```python
from build123d import *

# Parameters (mm, degrees)
BOSS_EXTRUDE1_DEPTH = 45
FILLET1_R           = 20
BOSS_EXTRUDE2_DEPTH = 19
BOSS_EXTRUDE3_DEPTH = 10
CUT_EXTRUDE2_REACH  = 92.422
SKETCH4_R           = 10
SKETCH4_R_2         = 5
SKETCH4_R_3         = 3
BOSS_EXTRUDE4_START = -9.5
SKETCH7_R           = 10
SKETCH7_R_2         = 5
BOSS_EXTRUDE4_DEPTH = 9.5


with BuildPart() as part:
    # Sketch1 → Boss-Extrude1 (new body)
    with BuildSketch(Plane.XY):
        Polygon((-53.872058339, 0), (-53.872058339, 13), (46.127941661, 13), (46.127941661, -4.908485857), (9.127941661, -4.908485857), (9.127941661, 0), align=None)
    extrude(amount=-BOSS_EXTRUDE1_DEPTH)

    # Fillet1
    fillet1_edges = [part.edges().sort_by_distance(p)[0] for p in [
        (46.127941661, 4.045757072, 0),
    ]]
    fillet(fillet1_edges, radius=FILLET1_R)

    # Sketch2 → Boss-Extrude2 (add)
    with BuildSketch(Plane(origin=(0, 0, -45), x_dir=(-1, 0, 0), z_dir=(0, 0, -1))):
        with BuildLine():
            Line((53.872058339, 13), (53.872058339, 51))
            ThreePointArc((53.872058339, 51), (34.872058339, 70), (15.872058339, 51))
            Line((15.872058339, 51), (15.872058339, 13))
            Line((15.872058339, 13), (53.872058339, 13))
        make_face()
        with BuildLine():
            Line((42.372058339, 51), (42.372058339, 32))
            ThreePointArc((42.372058339, 32), (34.872058339, 24.5), (27.372058339, 32))
            Line((27.372058339, 32), (27.372058339, 51))
            ThreePointArc((27.372058339, 51), (34.872058339, 58.5), (42.372058339, 51))
        make_face(mode=Mode.SUBTRACT)
    extrude(amount=-BOSS_EXTRUDE2_DEPTH)

    # Sketch3 → Boss-Extrude3 (add)
    with BuildSketch(Plane(origin=(0, 0, -45), x_dir=(-1, 0, 0), z_dir=(0, 0, -1))):
        Polygon((-46.127941661, 13), (16.803506509, 13), (18.329411345, 13), (18.329411345, 60.345631624), align=None)
    extrude(amount=-BOSS_EXTRUDE3_DEPTH)

    # Sketch4 → Cut-Extrude2 (cut, up to next)
    with BuildSketch(Plane(origin=(0, 13, 0), x_dir=(1, 0, 0), z_dir=(0, 1, 0)), mode=Mode.PRIVATE) as cut_extrude2_sk1:
        with Locations(Location((26.127941661, 20, 0), (0, 0, 270))):
            Circle(SKETCH4_R)
        with Locations((26.127941661, 20)):
            Circle(SKETCH4_R_2, mode=Mode.SUBTRACT)
    cut_extrude2_tool1 = extrude(cut_extrude2_sk1.sketch, amount=-CUT_EXTRUDE2_REACH, mode=Mode.PRIVATE) & part.part
    # Sketch4 → Cut-Extrude2 (cut, up to next)
    with BuildSketch(Plane(origin=(0, 13, 0), x_dir=(1, 0, 0), z_dir=(0, 1, 0)), mode=Mode.PRIVATE) as cut_extrude2_sk2:
        with Locations((26.127941661, 20)):
            Circle(SKETCH4_R_2)
        with Locations((26.127941661, 20)):
            Circle(SKETCH4_R_3, mode=Mode.SUBTRACT)
    cut_extrude2_tool2 = extrude(cut_extrude2_sk2.sketch, amount=-CUT_EXTRUDE2_REACH, mode=Mode.PRIVATE) & part.part
    # Sketch4 → Cut-Extrude2 (cut, up to next)
    with BuildSketch(Plane(origin=(0, 13, 0), x_dir=(1, 0, 0), z_dir=(0, 1, 0)), mode=Mode.PRIVATE) as cut_extrude2_sk3:
        with Locations((26.127941661, 20)):
            Circle(SKETCH4_R_3)
    cut_extrude2_tool3 = extrude(cut_extrude2_sk3.sketch, amount=-CUT_EXTRUDE2_REACH, mode=Mode.PRIVATE) & part.part
    add(cut_extrude2_tool1.solids().sort_by_distance((26.127942, 13, -29.717157))[0], mode=Mode.SUBTRACT)
    add(cut_extrude2_tool2.solids().sort_by_distance((21.269363, 13, -20))[0], mode=Mode.SUBTRACT)
    add(cut_extrude2_tool3.solids().sort_by_distance((26.127942, 13, -20))[0], mode=Mode.SUBTRACT)

    # Sketch7 → Boss-Extrude4 (add)
    with BuildSketch(Plane.XZ.offset(4.908485857).offset(BOSS_EXTRUDE4_START)):
        with Locations(Location((26.127941661, -20, 0), (0, 0, 90))):
            Circle(SKETCH7_R)
        with Locations((26.127941661, -20)):
            Circle(SKETCH7_R_2, mode=Mode.SUBTRACT)
    extrude(amount=BOSS_EXTRUDE4_DEPTH)


solid = part.part
```
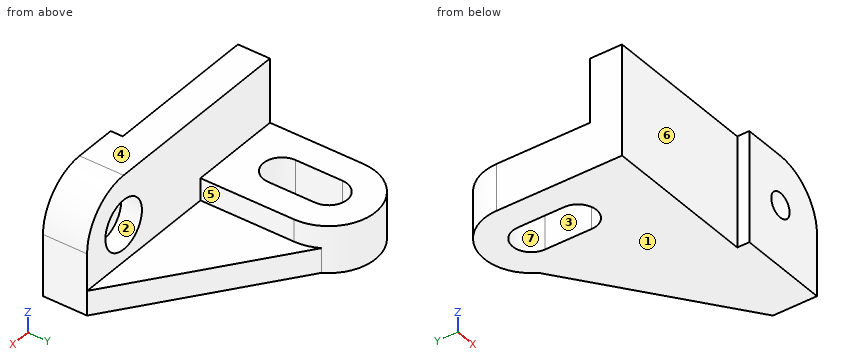
CAD build for the part. Positions are in the model's coordinates, mm. Face numbers are marked on the shaded views. A direction names the side the tool comes from. Round coordinates to 2 decimals unless told otherwise and drop trailing zeros. Loops run counter-clockwise (first coordinate to the right, second up) from the corner with the lowest first, then second, coordinate; pieces in that order, holes last. Notation, with made-up numbers: M -5.75,-38 L 3.25,-38 A21 ccw 3.25,-26 Z; hole C 3.25,-35.5 d7. An arc over 180 degrees is marked long. Use a Markdown table: item, result. Add a question column.
(1) Flat gauge pins, fed straight in: pin 1 (19 mm diameter, centred on x = -30, y = 52, fed in from +Z); pin 2 (1.5 mm diameter, centred on x = 35, y = 12, fed in from +Z); pin 3 (14 mm diameter, centred on x = 0, y = 27, fed in from +Z); pin 4 (1.5 mm diameter, centred on x = 31, y = 27, fed in from -Z). Where does each tip first touch, or does it go through?
(2) Drill centre lines: line 1 (X direction, y = 39, z = -29); line 2 (Y direction, x = -31.5, z = -8.5); line 3 (Z direction, x = -30.5, y = 24.5). Where is each one in solid material? Low to high.
(3) Cut at C-C (z = -38). Give the cut face in (x, y), and give its area (3 significant figures).
(4) Cut at D-D (y = 2). Give the cut face in (x, z).
(5) Which spindle directions (+Z, -Z, +X, -X, +Y, -Y) get a long thin tool onto all of the face, cutting with end or side? Do the marked faces 5, 6 and 7. Say none if no direction does.
(6) Pull direction Z, two halves, no side cores. Call the marked faces 1, 2, 3 and 4: +Z half, -Z half, draft (parallel to the pull), parting line (faces both ways), or undercut.
(7) Cut at A-A (x = -40). Give the cut face in (y, z), and give its area (3 significant figures).
(8) Cut at B-B (y = 53.5). Give the cut face in (x, z), and give its area (3 significant figures).
Geometry says:
| question | item | result |
|---|---|---|
| 1 | pin 1 | stops at z = -26 |
| 1 | pin 2 | stops at z = -1.72 |
| 1 | pin 3 | stops at z = -35 |
| 1 | pin 4 | passes through |
| 2 | line 1 | x = -53.87 to -42.37, -27.37 to -15.87 |
| 2 | line 2 | y = 0 to 13 |
| 2 | line 3 | z = -45 to -26 |
| 3 | outline | M -53.87,0 L 9.13,0 L 9.13,-4.91 L 46.13,-4.91 L 46.13,13 L -18.33,60.35 A19 ccw -53.87,51 Z; hole M -42.37,32 A7.5 ccw -27.37,32 L -27.37,51 A7.5 ccw -42.37,51 Z |
| 3 | area | 4,450 mm² |
| 4 | outline | M -53.87,-45 L 46.13,-45 L 46.13,-20 A20 ccw 26.13,0 L -53.87,0 Z; hole C 26.13,-20 d10 |
| 5 | face 5 | +Z, +X, +Y |
| 5 | face 6 | +Z, -Z, -X, -Y |
| 5 | face 7 | +Z, -Z |
| 6 | face 1 | -Z half |
| 6 | face 2 | undercut |
| 6 | face 3 | draft |
| 6 | face 4 | +Z half |
| 7 | outline | M 0,-45 L 26.53,-45 L 26.53,-26 L 13,-26 L 13,0 L 0,0 Z; M 56.47,-45 L 69.29,-45 L 69.29,-26 L 56.47,-26 Z |
| 7 | area | 1,090 mm² |
| 8 | outline | M -53.71,-45 L -41.94,-45 L -41.94,-26 L -53.71,-26 Z; M -27.8,-45 L -9.01,-45 L -9.01,-35 L -16.04,-35 L -16.04,-26 L -27.8,-26 Z |
| 8 | area | 517 mm² |
